For this review, use the dimensioned drawing (mm, ordinates from the lowest corner) and the shaded views. Round coordinates to 2 decimals unless told otherwise and drop trailing zeros. Loops run counter-clockwise (first coordinate to the right, second up) from the corner with the lowest first, then second, coordinate; pieces in that order, holes last.
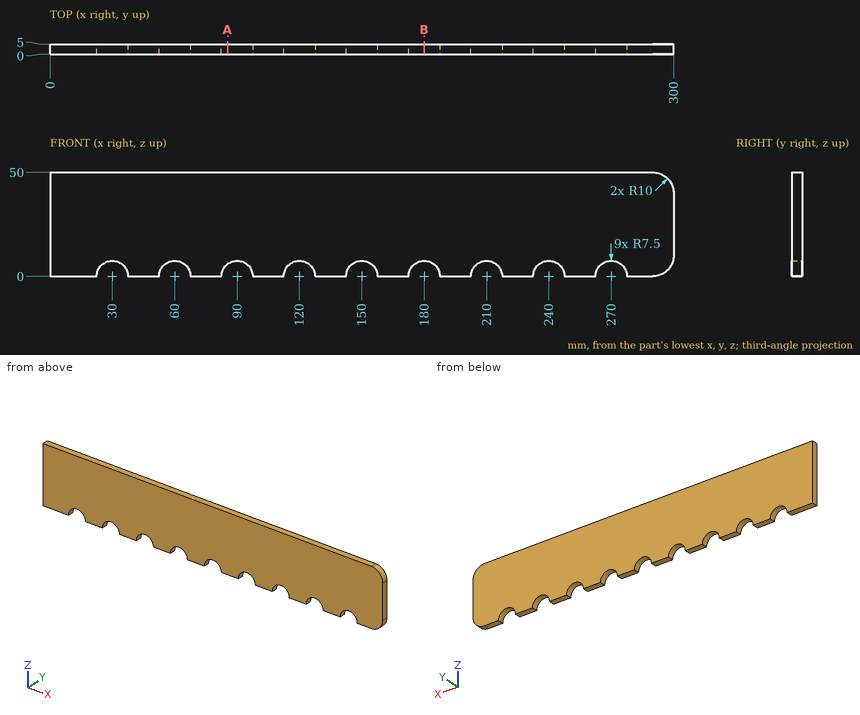
(1) Add section A-A (x = 85.5). Give the boundary of the cut face in (y, z), plus the area to 3 significant figures.
(2) Insertion check: pin 1 Ø2 at (x, y) = (61, 1.5) entering from -Z. The pin has a flat end and moves straight along its axis. Give the tip position at first contact, or say it passes through.
(3) Add section B-B (x = 180). Give the boundary of the cut face in (y, z), plus the area to 4 significant figures.
(4) For L1, parallel to X at y = 2.55, z = 41; L2, parallel to Z at x = 264, y = 2; L3, parallel to Z at x = 152.5, y = 4.45, list the stretches that pass through material, from the lowest coordinate up.
Outcome:
1. outline: (0, 6) - (5, 6) - (5, 50) - (0, 50) - close
1. area: 220 mm2
2. pin 1: stops at z = 7.23
3. outline: (0, 7.5) - (5, 7.5) - (5, 50) - (0, 50) - close
3. area: 212.5 mm2
4. L1: x = 0 to 299.95
4. L2: z = 4.5 to 50
4. L3: z = 7.07 to 50
